Here's how the part is built. I have some questions about the finished solid (model axes, mm). A direction names the side the tool comes from. Round coordinates to 2 decimals unless told otherwise and drop trailing zeros. Write each loop counter-clockwise with the first axis right and the second up, starting at its lowest first coordinate (ties: lowest second). Pieces come first, ordered by that corner, then holes. Notation, with made-up numbers: (-32, -18.75) - (18, -18.75) arc R33 ccw to (18, 11.25) - close; hole circle Ø8 at (12.25, 29). An arc over 180 degrees is marked (long way). Use one line per item in the form item = value. Start each with the question number.
1. Which directions (+Z, -Z, +X, -X, +Y, -Y) give clear straight access to the entire face, cutting with the end or side of a thin tool? Please do faces 1 (the cylindrical face through (46.186, -168.246, -1.197)), 2 (the flat face through (49, -154.045, 3)), 3 (the cylindrical face through (-43.984, -168.246, -1.197)).
2. I want a section at C-C, the plane z = 1.5. List the corners of the cut face in (x, y) for me, plus the area to 3 significant figures.
3. I want a section at A-A, the plane y = -138. List the corners of the cut face in (x, z) for me, plus the area to 3 significant figures.
4. We'd pull the mould along X, two halves only. Please class faces 4 (the flat face through (-49.69, -129, 1)), 5 (the flat face through (-46, -154.045, 3)), 6 (the flat face through (13, -132, 5.08)): +X half, -X half, draft (parallel to the pull), parting line (faces both ways), or undercut.
5. Will these pins go through, and if not, where does the flat tip stop? pin 1 (1.5 mm diameter, centred on x = 48, z = 1.5, fed in from -Y); pin 2 (4 mm diameter, centred on x = -36.5, y = -164, fed in from -Z); pin 3 (6 mm diameter, centred on x = -6, y = -151.5, fed in from -Z); pin 4 (12 mm diameter, centred on x = 39, y = -122.5, fed in from +Z).
6. If I drill on line 1 along Z through (x, y) = (-6, -157.5); line 2 along Y through (x, z) = (-19, 4); line 3 along X through (y, z) = (-119.5, 4.25), over which ranges is the centre line in solid material (lowest first)?
7. I want a section at B-B, the plane x = 12. List the corners of the cut face in (y, z) for me, plus the area to 3 significant figures.
8. I want a section at D-D, the plane x = 32.5. List the corners of the cut face in (y, z) for me, plus the area to 3 significant figures.
```python
from build123d import *

# Parameters (mm, degrees)
EXTRUDE1_DEPTH               = 5.08
FILLET1_R                    = 2.54
CHAMFER1_SIZE2               = 5.08
CHAMFER1_SIZE                = 8.798818102
EXTRUDE3_DEPTH               = 88.9
EXTRUDE4_DEPTH               = 0.762
SALIENTE_EXTRUIR1_DEPTH      = 1.27
SALIENTE_EXTRUIR1_DEPTH_BACK = 90.17
SKETCH2_R                    = 1.003990475


with BuildPart() as part:
    # Sketch1 → Extrude1 (new body)
    with BuildSketch(Plane.XY):
        Polygon((-49.690313901, -102.787097767), (51.909686099, -102.787097767), (51.909686099, -154.045409896), (45.559686099, -154.045409896), (45.559686099, -170.008151162), (-43.340313901, -170.008151162), (-43.340313901, -154.045409896), (-49.690313901, -154.045409896), align=None)
    extrude(amount=EXTRUDE1_DEPTH)

    # Fillet1
    fillet1_edges = [part.edges().sort_by_distance(p)[0] for p in [
        (51.909686099, -128.416253832, 5.08),
        (-49.690313901, -128.416253832, 5.08),
    ]]
    fillet(fillet1_edges, radius=FILLET1_R)

    # Chamfer1
    chamfer1_edges = [part.edges().sort_by_distance(p)[0] for p in [
        (1.109686099, -170.008151162, 5.08),
    ]]
    chamfer1_side = [part.faces().sort_by_distance(p)[0] for p in [
        (1.109686099, -169.906551162, 5.08),
    ]]
    chamfer(chamfer1_edges, length=CHAMFER1_SIZE - 0.0001, length2=CHAMFER1_SIZE2 - 0.0001, reference=chamfer1_side[0])  # a hair under: the kernel refuses the full size

    # Sketch3 → Extrude3 (add)
    with BuildSketch(Plane(origin=(45.559686099, 0, 0), x_dir=(0, 0, -1), z_dir=(1, 0, 0))):
        with BuildLine():
            Line((-2.656143456, -165.407575745), (0, -170.008151162))
            ThreePointArc((0, -170.008151162), (2.094834297, -170.56946032), (2.656143456, -168.474626023))
            Line((2.656143456, -168.474626023), (0, -163.874050605))
            Line((0, -163.874050605), (-2.656143456, -165.407575745))
        make_face()
    extrude(amount=-EXTRUDE3_DEPTH)

    # Sketch4 → Extrude4 (add)
    with BuildSketch(Plane.XY.offset(5.08)):
        with BuildLine():
            Line((2.697186099, -113.368491021), (2.697186099, -140.858908158))
            ThreePointArc((2.697186099, -140.858908158), (1.109686099, -142.446408158), (-0.477813901, -140.858908158))
            Line((-0.477813901, -140.858908158), (-0.477813901, -113.368491021))
            ThreePointArc((-0.477813901, -113.368491021), (1.109686099, -111.780991021), (2.697186099, -113.368491021))
        make_face()
        with BuildLine():
            Line((-31.531803629, -113.368491021), (-31.531803629, -140.858908158))
            ThreePointArc((-31.531803629, -140.858908158), (-29.944303629, -142.446408158), (-28.356803629, -140.858908158))
            Line((-28.356803629, -140.858908158), (-28.356803629, -113.368491021))
            ThreePointArc((-28.356803629, -113.368491021), (-29.944303629, -111.780991021), (-31.531803629, -113.368491021))
        make_face()
        with BuildLine():
            Line((33.751175827, -113.368491021), (33.751175827, -140.858908158))
            ThreePointArc((33.751175827, -140.858908158), (32.163675827, -142.446408158), (30.576175827, -140.858908158))
            Line((30.576175827, -140.858908158), (30.576175827, -113.368491021))
            ThreePointArc((30.576175827, -113.368491021), (32.163675827, -111.780991021), (33.751175827, -113.368491021))
        make_face()
    extrude(amount=EXTRUDE4_DEPTH)

    # Sketch2 → Saliente-Extruir1 (add, two sides: drawn at the far end of the back side and taken through both)
    with BuildSketch(Plane(origin=(45.559686099, 0, 0), x_dir=(0, 0, -1), z_dir=(1, 0, 0)).offset(-SALIENTE_EXTRUIR1_DEPTH_BACK)):
        with Locations((1.328071728, -169.241388592)):
            Circle(SKETCH2_R)
    extrude(amount=SALIENTE_EXTRUIR1_DEPTH + SALIENTE_EXTRUIR1_DEPTH_BACK)


solid = part.part
```
Model answer:
q1.face_1 = +X
q1.face_2 = +Z, -Z, +X, -Y
q1.face_3 = -X
q2.outline = (-49.69, -154.05) - (-43.34, -154.05) - (-43.34, -167.41) - (45.56, -167.41) - (45.56, -154.05) - (51.91, -154.05) - (51.91, -102.79) - (-49.69, -102.79) - close
q2.area = 6,400 mm2
q3.outline = (-49.69, 0) - (51.91, 0) - (51.91, 2.54) arc R2.54 ccw to (49.37, 5.08) - (33.75, 5.08) - (33.75, 5.84) - (30.58, 5.84) - (30.58, 5.08) - (2.7, 5.08) - (2.7, 5.84) - (-0.48, 5.84) - (-0.48, 5.08) - (-28.36, 5.08) - (-28.36, 5.84) - (-31.53, 5.84) - (-31.53, 5.08) - (-47.15, 5.08) arc R2.54 ccw to (-49.69, 2.54) - close
q3.area = 521 mm2
q4.face_4 = -X half
q4.face_5 = draft
q4.face_6 = undercut
q5.pin_1 = -154.05
q5.pin_2 = -1.23
q5.pin_3 = 0
q5.pin_4 = 5.84
q6.line_1 = 0 to 5.08
q6.line_2 = -163.08 to -102.79
q6.line_3 = -49.03 to 51.25
q7.outline = (-170.01, 0) arc R1.53 ccw to (-168.47, -2.66) - (-163.87, 0) - (-102.79, 0) - (-102.79, 5.08) - (-161.21, 5.08) - close
q7.area = 331 mm2
q8.outline = (-170.01, 0) arc R1.53 ccw to (-168.47, -2.66) - (-163.87, 0) - (-102.79, 0) - (-102.79, 5.08) - (-111.82, 5.08) - (-111.82, 5.84) - (-142.41, 5.84) - (-142.41, 5.08) - (-161.21, 5.08) - close
q8.area = 354 mm2
